Source: CAD feature listing. Evaluate the final solid. Frame: model axes, mm. Round coordinates to 2 decimals unless told otherwise and drop trailing zeros. Loops run counter-clockwise (first coordinate to the right, second up) from the corner with the lowest first, then second, coordinate; pieces in that order, holes last.
Item 1: Pull-direction query (X, two-part tool) for faces 1 (the cylindrical face through (336.793, 1.61, -76.225)), 2 (the flat face through (414, 3.175, -258)); classes: released by +X, released by -X, zero draft, split by the parting line, or undercut.
Item 2: Section query A-A on x = 328.5. Return loops of the section in (y, z) (3 decimals).
Item 3: Ray query, L1, parallel to Z at x = 444.5, y = 1.1; L2, parallel to Z at x = 330.2, y = 1.8; L3, parallel to X at y = 0.8, z = -88.9. Return the intervals inside material, ascending.
```python
from build123d import *

# Parameters (mm, degrees)
SKETCH1_W               = 571.5
SKETCH1_H               = 508
BOSS_EXTRUDE1_DEPTH     = 3.175
SKETCH2_R               = 14.2875
CUT_EXTRUDE1_DEPTH      = 3.175
SKETCH4_R               = 2.0193
CUT_EXTRUDE3_DEPTH      = 1
CUT_EXTRUDE3_DEPTH_BACK = 4.175
SKETCH5_W               = 619.579537293
SKETCH5_H               = 89.035098343
CUT_EXTRUDE4_DEPTH      = 165.1
SKETCH6_W               = 508
SKETCH6_H               = 3.175
CUT_EXTRUDE5_DEPTH      = 96.52


with BuildPart() as part:
    # Sketch1 → Boss-Extrude1 (new body)
    with BuildSketch(Plane(origin=(0, 0, 0), x_dir=(1, 0, 0), z_dir=(0, 1, 0))):
        with Locations((285.75, 254)):
            Rectangle(SKETCH1_W, SKETCH1_H)
    extrude(amount=BOSS_EXTRUDE1_DEPTH)

    # Sketch2 → Cut-Extrude1 (cut)
    with BuildSketch(Plane(origin=(0, 3.175, 0), x_dir=(1, 0, 0), z_dir=(0, 1, 0))):
        with Locations((330.2, 419.1)):
            Circle(SKETCH2_R)
        with Locations((330.2, 88.9)):
            Circle(SKETCH2_R)
    extrude(amount=-CUT_EXTRUDE1_DEPTH, mode=Mode.SUBTRACT)

    # Sketch4 → Cut-Extrude3 (cut, two sides)
    with BuildSketch(Plane(origin=(0, 3.175, 0), x_dir=(1, 0, 0), z_dir=(0, 1, 0))) as cut_extrude3_sk:
        with Locations((546.1, 495.3)):
            Circle(SKETCH4_R)
        with Locations((520.7, 495.3)):
            Circle(SKETCH4_R)
        with Locations((495.3, 495.3)):
            Circle(SKETCH4_R)
        with Locations((469.9, 495.3)):
            Circle(SKETCH4_R)
        with Locations((444.5, 495.3)):
            Circle(SKETCH4_R)
        with Locations((419.1, 495.3)):
            Circle(SKETCH4_R)
        with Locations((393.7, 495.3)):
            Circle(SKETCH4_R)
        with Locations((368.3, 495.3)):
            Circle(SKETCH4_R)
        with Locations((342.9, 495.3)):
            Circle(SKETCH4_R)
        with Locations((317.5, 495.3)):
            Circle(SKETCH4_R)
        with Locations((292.1, 495.3)):
            Circle(SKETCH4_R)
        with Locations((266.7, 495.3)):
            Circle(SKETCH4_R)
        with Locations((228.6, 495.3)):
            Circle(SKETCH4_R)
        with Locations((203.2, 495.3)):
            Circle(SKETCH4_R)
        with Locations((203.2, 12.7)):
            Circle(SKETCH4_R)
        with Locations((228.6, 12.7)):
            Circle(SKETCH4_R)
        with Locations((266.7, 12.7)):
            Circle(SKETCH4_R)
        with Locations((292.1, 12.7)):
            Circle(SKETCH4_R)
        with Locations((317.5, 12.7)):
            Circle(SKETCH4_R)
        with Locations((342.9, 12.7)):
            Circle(SKETCH4_R)
        with Locations((368.3, 12.7)):
            Circle(SKETCH4_R)
        with Locations((393.7, 12.7)):
            Circle(SKETCH4_R)
        with Locations((419.1, 12.7)):
            Circle(SKETCH4_R)
        with Locations((444.5, 12.7)):
            Circle(SKETCH4_R)
        with Locations((469.9, 12.7)):
            Circle(SKETCH4_R)
        with Locations((495.3, 12.7)):
            Circle(SKETCH4_R)
        with Locations((520.7, 12.7)):
            Circle(SKETCH4_R)
        with Locations((546.1, 12.7)):
            Circle(SKETCH4_R)
    extrude(amount=CUT_EXTRUDE3_DEPTH, mode=Mode.SUBTRACT)
    extrude(cut_extrude3_sk.sketch, amount=-CUT_EXTRUDE3_DEPTH_BACK, mode=Mode.SUBTRACT)

    # Sketch5 → Cut-Extrude4 (cut)
    with BuildSketch(Plane.ZY):
        with Locations((-257.641209254, 26.710529503)):
            Rectangle(SKETCH5_W, SKETCH5_H)
    extrude(amount=-CUT_EXTRUDE4_DEPTH, mode=Mode.SUBTRACT)

    # Sketch6 → Cut-Extrude5 (cut)
    with BuildSketch(Plane.ZY.offset(-165.1)):
        with Locations((-254, 1.5875)):
            Rectangle(SKETCH6_W, SKETCH6_H)
    extrude(amount=-CUT_EXTRUDE5_DEPTH, mode=Mode.SUBTRACT)


solid = part.part
```
Data:
1. face 1: undercut
1. face 2: zero draft
2. outline: (0, -508) - (3.175, -508) - (3.175, -433.286) - (0, -433.286) - close; (0, -404.914) - (3.175, -404.914) - (3.175, -103.086) - (0, -103.086) - close; (0, -74.714) - (3.175, -74.714) - (3.175, 0) - (0, 0) - close
3. L1: z = -508 to -497.32, -493.28 to -14.72, -10.68 to 0
3. L2: z = -508 to -433.39, -404.81 to -103.19, -74.61 to 0
3. L3: x = 261.62 to 315.91, 344.49 to 571.5
